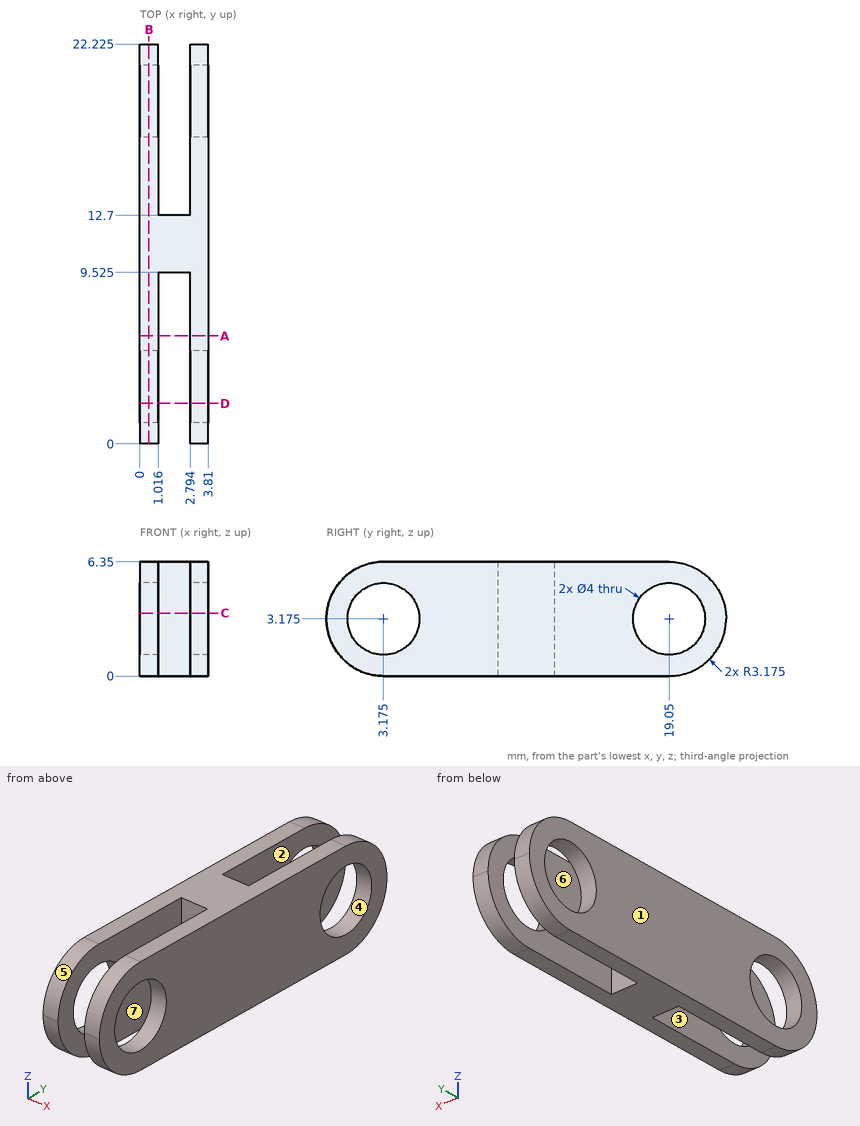
Here's the drawing with two shaded views (mm, measured from the low corner). I have some questions. A direction names the side the tool comes from. Coordinates: 2 decimals unless noted, no trailing zeros. Order: outer loops, then holes, each group sorted by start corner. A loop starts at its lowest first (then second) coordinate and runs counter-clockwise, first axis right, second up.
Item 1: I need wall thicknesses on line 1 (Z direction, x = 0.3, y = 19.05) (3 decimals); line 2 (X direction, y = 8.75, z = 5.75); line 3 (Y direction, x = 3, z = 4). Which ranges of each line are inside material? Lowest first, please.
Result sheet:
line 1: z = 0 to 1.175, 5.175 to 6.35
line 2: x = 0 to 1.02, 2.79 to 3.81
line 3: y = 0.11 to 1.35, 5 to 17.23, 20.87 to 22.12
Item 2: If we mould it in two halves opening along X, with no side actions, what happens to the marked faces 1, 2, 3 and 4? For each: +X half, -X half, draft (parallel to the pull), parting line (faces both ways), or undercut.
Result sheet:
face 1: -X half
face 2: undercut
face 3: undercut
face 4: draft
Item 3: If we section it at C-C on z = 3.5: List the corners of the cut face in (x, y) for me (3 decimals).
Result sheet:
outline: (0, 0.017) - (1.016, 0.017) - (1.016, 1.202) - (0, 1.202) - close; (0, 5.148) - (1.016, 5.148) - (1.016, 9.525) - (2.794, 9.525) - (2.794, 5.148) - (3.81, 5.148) - (3.81, 17.077) - (2.794, 17.077) - (2.794, 12.7) - (1.016, 12.7) - (1.016, 17.077) - (0, 17.077) - close; (0, 21.023) - (1.016, 21.023) - (1.016, 22.208) - (0, 22.208) - close; (2.794, 0.017) - (3.81, 0.017) - (3.81, 1.202) - (2.794, 1.202) - close; (2.794, 21.023) - (3.81, 21.023) - (3.81, 22.208) - (2.794, 22.208) - close
Item 4: If we section it at D-D on y = 2.25: List the corners of the cut face in (x, z) for me.
Result sheet:
outline: (0, 0.14) - (1.02, 0.14) - (1.02, 1.4) - (0, 1.4) - close; (0, 4.95) - (1.02, 4.95) - (1.02, 6.21) - (0, 6.21) - close; (2.79, 0.14) - (3.81, 0.14) - (3.81, 1.4) - (2.79, 1.4) - close; (2.79, 4.95) - (3.81, 4.95) - (3.81, 6.21) - (2.79, 6.21) - close
Item 5: If we section it at A-A on y = 6: List the corners of the cut face in (x, z) for me, plus the area to 3 significant figures.
Result sheet:
outline: (0, 0) - (1.02, 0) - (1.02, 6.35) - (0, 6.35) - close; (2.79, 0) - (3.81, 0) - (3.81, 6.35) - (2.79, 6.35) - close
area: 12.9 mm2
Item 6: For P1, Ø1.4, axis at x = 2, z = 4.5, coming from the +Y side; P2, Ø0.5, axis at x = 2, z = 4, coming from the -Y side (3 decimals), each with a flat end and sliding along its axis, tell me the tip position at first contact or that it passes through.
Result sheet:
P1: stops at y = 12.7
P2: stops at y = 9.525
Item 7: For the marked faces 5, 6 and 7, which set-ups out of +Z, -Z, +X, -X, +Y, -Y let a thin tool reach every point of the face, with its end or its side?
Result sheet:
face 5: +Z, +X, -X, -Y
face 6: +Z, -Z, +Y
face 7: +Z, -Z, -Y
Item 8: If we section it at B-B on x = 0.5: State how many separate pieces and enclosed holes the cut face has, plus the area to 3 significant figures.
Result sheet:
separate pieces: 1
enclosed holes: 2
area: 107 mm2
